Verification items for this drawing (mm, ordinates from the low corner). A direction names the side the tool comes from. Give positions to 0.01 mm unless a question says otherwise; leave off trailing zeros. Loops run counter-clockwise (first coordinate to the right, second up) from the corner with the lowest first, then second, coordinate; pieces in that order, holes last. Notation, with made-up numbers: M 30.25,42.25 L 84.25,42.25 A26 ccw 84.25,69.25 Z; hole C 46.5,-17.5 d2. An arc over 180 degrees is marked long. Answer in a Markdown table with one row per item.
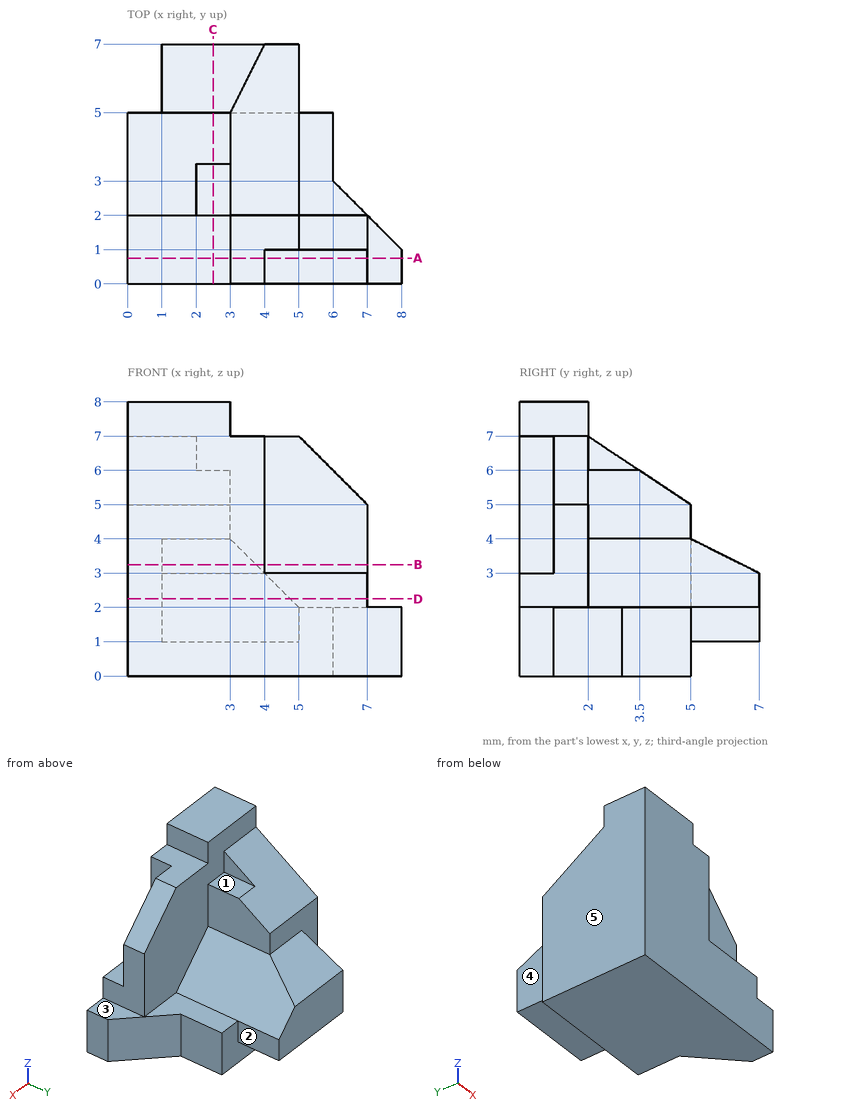
Item 1: Scan lines: L1, parallel to X at y = 2, z = 0.5; L2, parallel to Y at x = 6.5, z = 3.5; L3, parallel to X at y = 2.5, z = 6.5. Record each from-to range of solid material in increasing order. Write a range as [from, to].
Reported:
| item | result |
|---|---|
| L1 | x = [0, 7] |
| L2 | y = [1, 2] |
| L3 | x = [0, 2] |
Item 2: Go/stop test with flat-tipped pins: pin 1 (0.5 mm diameter, centred on y = 3, z = 6.5, fed in from +X); pin 2 (1.1 mm diameter, centred on y = 0.5, z = 5, fed in from +X); pin 3 (0.6 mm diameter, centred on x = 6, y = 3, fed in from +Z). Record where each tip stops, or that it passes through.
Reported:
| item | result |
|---|---|
| pin 1 | stops at x = 2 |
| pin 2 | stops at x = 7 |
| pin 3 | stops at z = 2 |
Item 3: Sectioned sample at A-A (y = 0.75). Record the cut outline in (x, z), and give its area (3 significant figures).
Reported:
| item | result |
|---|---|
| outline | M 0,0 L 8,0 L 8,2 L 7,2 L 7,3 L 4,3 L 4,7 L 3,7 L 3,8 L 0,8 Z |
| area | 42.0 mm^2 |
Item 4: Sectioned sample at D-D (z = 2.25). Record the cut outline in (x, y), and give its area (4 significant figures).
Reported:
| item | result |
|---|---|
| outline | M 0,0 L 7,0 L 7,2 L 4.75,2 L 4.75,7 L 1,7 L 1,5 L 0,5 Z |
| area | 35.75 mm^2 |
Item 5: Sectioned sample at C-C (x = 2.5). Record the cut outline in (y, z).
Reported:
| item | result |
|---|---|
| outline | M 0,0 L 5,0 L 5,1 L 7,1 L 7,3 L 5,4 L 5,5 L 3.5,6 L 2,6 L 2,8 L 0,8 Z |
Item 6: Sectioned sample at B-B (z = 3.25). Record the cut outline in (x, y).
Reported:
| item | result |
|---|---|
| outline | M 0,0 L 4,0 L 4,1 L 7,1 L 7,2 L 3.75,2 L 3.75,6.5 L 1,6.5 L 1,5 L 0,5 Z |
Item 7: Tool access check on the marked faces 1, 2, 3, 4 and 5. Record the directions out of +Z, -Z, +X, -X, +Y, -Y that give a thin tool (end or side, any length) a straight path to the whole face; none if there is none.
Reported:
| item | result |
|---|---|
| face 1 | +Z, +X, +Y |
| face 2 | +Z, -Z, +X, +Y |
| face 3 | +Z, +X, +Y, -Y |
| face 4 | +Z, -Z, -X, +Y |
| face 5 | +Z, -Z, -X, +Y, -Y |
